The model under review builds one solid part; all positions refer to its coordinate system, in mm. A direction names the side the tool comes from. Give positions to 0.01 mm unless a question says otherwise; leave off trailing zeros. Loops run counter-clockwise (first coordinate to the right, second up) from the corner with the lowest first, then second, coordinate; pieces in that order, holes last. Notation, with made-up numbers: (-9, 27.25) -> (10, 27.25) arc R15 cw to (10, 43.25) -> close; hole circle Ø6 at (7, 21.25). An arc over 180 degrees is marked (long way). Write each question's results on one line, items separated by ' | '. Start each with the question number.
Q1. We need section C-C (z = 0). Write out the cut boundary in (x, y), plus the area to 3 significant figures.
Q2. We need section A-A (y = 1.75). Write out the cut boundary in (x, z), plus the area to 3 significant figures.
Q3. Insertion check: pin 1 Ø4 at (x, z) = (1, -1) entering from +Y; pin 2 Ø0.9 at (x, z) = (2.5, 3) entering from +Y; pin 3 Ø1 at (x, y) = (-0.5, 4) entering from -Z. Each pin has a flat end and moves straight along its axis. Give the tip position at first contact, or say it passes through.
Q4. Machinability: for faces 5 (the face through (-1.49, 2.46, 3.2)), 6 (the face through (0.54, 3.99, 2.44)), which of the approach directions +Z, -Z, +X, -X, +Y, -Y give a long, thin tool a straight path to every point of the face, cutting with its end or side? Answer none if there is none.
Q5. Wall thickness on L1, parallel to Y at x = 1.75, z = 0.75; L2, parallel to Z at x = 0, y = 4.5; L3, parallel to X at y = 3.7, z = 2: over which ranges is each line inside the solid? List them lowest first. Write a range as [from, to].
Q6. We need section B-B (y = 4.2). Write out the cut boundary in (x, z), plus the area to 3 significant figures.
Q7. Mouldability with a two-part tool opening along Z and no side actions: class faces 1 (the face through (4.37, 3.99, 4.09)), 2 (the face through (0, 3, 0)), 3 (the face through (-3, 2, -2)), 4 (the face through (5, 2, 2)) as released by +Z, released by -Z, zero draft, split by the parting line, or undercut.
Q8. We need section D-D (z = 2). Write out the cut boundary in (x, y).
Autodesk Inventor part; units mm, degrees
ref_plane "YZ Plane" through (0, 0, 0) normal (1, 0, 0) x (0, 1, 0)
ref_plane "XZ Plane" through (0, 0, 0) normal (0, 1, 0) x (-1, 0, 0)
ref_plane "XY Plane" through (0, 0, 0) normal (0, 0, 1) x (1, 0, 0)
sketch "Sketch1" plane through (0, 0, 0) normal (0, 1, 0) x (-1, 0, 0)
  line L0 (-0.4846, 5) -> (-5, 5)
  line L1 (-5, 5) -> (-5, -0.4418)
  line L2 (2.3844, 2.3844) -> (-2.6156, -2.6156) construction
  line L3 (-5, 5) -> (2.5, -2.5) construction
  circle A0 centre (0, 0) radius 2.5
  circle A1 centre (-3.1787, 3.1787) radius 1.5
  line L4 (-0.4846, 5) -> (5, 0)
  line L5 (5, 0) -> (0, -5)
  line L6 (0, -5) -> (-5, -0.4418)
  dimension "d2" = 5
  dimension "d3" = 3
extrude "Extrusion1" add sketch "Sketch1" along normal blind 5
sketch "Sketch2" plane through (0, 0, 0) normal (0, -1, 0) x (1, 0, 0)
  circle A0 centre (0, 0) radius 2.5
  circle A1 centre (3.1787, 3.1787) radius 1.5
extrude "Extrusion2" add sketch "Sketch2" against normal blind 3
chamfer "Chamfer1" distance 2 angle 45 2 edges at (0, 2.5, -5) (-5, 2.5, 0)
chamfer "Chamfer2" distance 0.5 angle 45 1 edges at (5, 2.5, 5)
properties part number "test_fit_3_5"
Output:
1) outline: (-3.55, 0) -> (5, 0) -> (5, 5) -> (2.5, 5) -> (2.5, 3) -> (-2.5, 3) -> (-2.5, 5) -> (-3.55, 5) -> close | area: 32.8 mm2
2) outline: (-3.59, -1.41) -> (-1.41, -3.59) -> (1.48, -3.65) -> (5, -0.44) -> (5, 4.5) -> (4.5, 5) -> (0.48, 5) -> (-3.52, 1.35) -> close | area: 58.3 mm2
3) pin 1: y = 5 | pin 2: y = 3 | pin 3: z = -3.62
4) face 5: +Z, -X, +Y, -Y | face 6: +Y
5) L1: [0, 3] | L2: [-3.62, -2.5], [2.5, 4.56] | L3: [-2.81, -1.5], [1.5, 2.25], [4.11, 5]
6) outline: (-3.59, -1.41) -> (-1.41, -3.59) -> (1.48, -3.65) -> (5, -0.44) -> (5, 4.5) -> (4.5, 5) -> (0.48, 5) -> (-3.52, 1.35) -> close; hole circle Ø5 at (0, 0); hole circle Ø3 at (3.18, 3.18) | area: 31.6 mm2
7) face 1: undercut | face 2: undercut | face 3: released by -Z | face 4: zero draft
8) outline: (-2.81, 0) -> (5, 0) -> (5, 5) -> (4.11, 5) -> (4.11, 3) -> (2.25, 3) -> (2.25, 5) -> (1.5, 5) -> (1.5, 3) -> (-1.5, 3) -> (-1.5, 5) -> (-2.81, 5) -> close
